Answer from the drawing. Dimensions are ordinates in mm from the lowest x, y and z of the part. Round coordinates to 2 decimals unless told otherwise and drop trailing zeros. Order: outer loops, then holes, each group sorted by start corner. A loop starts at its lowest first (then second) coordinate and runs counter-clockwise, first axis right, second up.
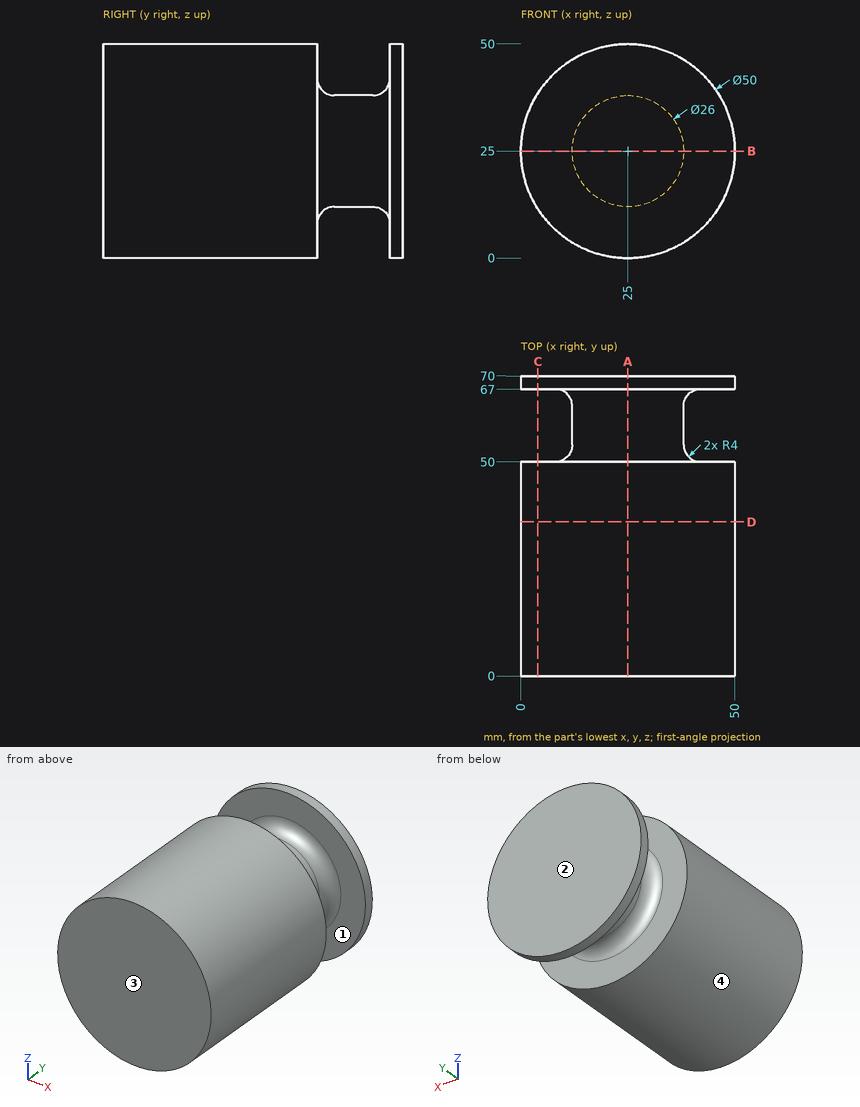
Q1. For a pull along Y with two mould halves and no side action, classify the marked faces 1, 2, 3 and 4 as released by +Y, released by -Y, zero draft, split by the parting line, or undercut.
Outcome:
face 1: undercut
face 2: released by +Y
face 3: released by -Y
face 4: zero draft
Q2. A cutting plane is placed at A-A, the plane x = 25. Give the vertices of the cut face in (y, z), plus the area to 3 significant figures.
Outcome:
outline: (0, 0) - (50, 0) - (50, 8) arc R4 cw to (54, 12) - (63, 12) arc R4 cw to (67, 8) - (67, 0) - (70, 0) - (70, 50) - (67, 50) - (67, 42) arc R4 cw to (63, 38) - (54, 38) arc R4 cw to (50, 42) - (50, 50) - (0, 50) - close
area: 3,110 mm2
Q3. A cutting plane is placed at B-B, the plane z = 25. Give the vertices of the cut face in (x, y), plus the area to 3 significant figures.
Outcome:
outline: (0, 0) - (50, 0) - (50, 50) - (42, 50) arc R4 cw to (38, 54) - (38, 63) arc R4 cw to (42, 67) - (50, 67) - (50, 70) - (0, 70) - (0, 67) - (8, 67) arc R4 cw to (12, 63) - (12, 54) arc R4 cw to (8, 50) - (0, 50) - close
area: 3,110 mm2
Q4. A cutting plane is placed at C-C, the plane x = 4. Give the vertices of the cut face in (y, z).
Outcome:
outline: (0, 11.44) - (50, 11.44) - (50, 38.56) - (0, 38.56) - close; (67, 11.44) - (70, 11.44) - (70, 38.56) - (67, 38.56) - close
Q5. A cutting plane is placed at D-D, the plane y = 36. Give the vertices of the cut face in (x, z), plus the area to 3 significant figures.
Outcome:
outline: circle Ø50 at (25, 25)
area: 1,960 mm2
Q6. Flat-ended cylindrical pins translate along their axes: pin 1 (2 mm diameter, centred on y = 49.5, z = 8, fed in from -X); pin 2 (10 mm diameter, centred on x = 7.5, y = 42.5, fed in from +Z); pin 3 (10 mm diameter, centred on x = 44.5, y = 27, fed in from +Z); pin 4 (5 mm diameter, centred on x = 41.5, y = 55.5, fed in from -Z). Find the tip coordinate at first contact, or state that the pin passes through.
Outcome:
pin 1: stops at x = 5.79
pin 2: stops at z = 46.65
pin 3: stops at z = 45.37
pin 4: passes through
Q7. Straight lines are drawn through the part: probe 1 along Y at (x, z) = (43, 27); probe 2 along Y at (x, z) = (20, 38.5); probe 3 along Z at (x, y) = (7.5, 34). For each, find the intervals that lie inside material, in ascending order.
Outcome:
probe 1: y = 0 to 50, 67 to 70
probe 2: y = 0 to 50.96, 66.04 to 70
probe 3: z = 7.15 to 42.85
